Read the model definition and answer for the solid it produces. Units are mm, in the model's axes. A direction names the side the tool comes from. Round coordinates to 2 decimals unless told otherwise and drop trailing zeros. Order: outer loops, then holes, each group sorted by start corner. A loop starts at its lowest first (then second) coordinate and runs counter-clockwise, first axis right, second up.
from build123d import *
from build123d.topology import SkipClean

# Parameters (mm, degrees)
SKETCH1_R               = 1.8
MOUNTING_FACE_DEPTH     = 7.5
CELL_SUPPORT_FILLETS_R  = 7.5
MIDLINE_START           = 5
SKETCH3_W               = 20
SKETCH3_H               = 6
SKETCH3_R               = 1.8
SKETCH3_W_2             = 8
SKETCH3_H_2             = 9
MIDLINE_EXTENSION_DEPTH = 5


with BuildPart() as part:
    # Sketch1 → Mounting Face (new body)
    with BuildSketch(Plane.XY):
        Polygon((130, 0), (130, 9), (81.25, 9), (81.25, 44), (51.25, 44), (51.25, 9), (0, 9), (0, 0), align=None)
        with Locations((4, 3)):
            Circle(SKETCH1_R, mode=Mode.SUBTRACT)
        with Locations((61.25, 3)):
            Circle(SKETCH1_R, mode=Mode.SUBTRACT)
        with Locations((71.25, 3)):
            Circle(SKETCH1_R, mode=Mode.SUBTRACT)
        with Locations((125.75, 3)):
            Circle(SKETCH1_R, mode=Mode.SUBTRACT)
    extrude(amount=MOUNTING_FACE_DEPTH)

    # Cell Support Fillets
    cell_support_fillets_edges = [part.edges().sort_by_distance(p)[0] for p in [
        (51.25, 9, 3.75),
        (81.25, 9, 3.75),
    ]]
    fillet(cell_support_fillets_edges, radius=CELL_SUPPORT_FILLETS_R)

    # Sketch3 → Midline Extension (add)
    # profile 1 of 3: a face of its own
    with SkipClean():  # the faces are left unmerged after this step: merging them gives an invalid solid
        with BuildSketch(Plane(origin=(0, 0, 0), x_dir=(-1, 0, 0), z_dir=(0, 0, -1)).offset(MIDLINE_START)):
            with Locations((-66.25, 3)):
                Rectangle(SKETCH3_W, SKETCH3_H)
            with Locations((-71.25, 3)):
                Circle(SKETCH3_R, mode=Mode.SUBTRACT)
            with Locations((-61.25, 3)):
                Circle(SKETCH3_R, mode=Mode.SUBTRACT)
        # profile 2 of 3: a face of its own
        with BuildSketch(Plane(origin=(0, 0, 0), x_dir=(-1, 0, 0), z_dir=(0, 0, -1)).offset(MIDLINE_START)):
            with Locations((-4, 4.5)):
                Rectangle(SKETCH3_W_2, SKETCH3_H_2)
            with Locations((-4, 3)):
                Circle(SKETCH3_R, mode=Mode.SUBTRACT)
        # profile 3 of 3: a face of its own
        with BuildSketch(Plane(origin=(0, 0, 0), x_dir=(-1, 0, 0), z_dir=(0, 0, -1)).offset(MIDLINE_START)):
            with BuildLine():
                Line((-130, 0), (-124, 0))
                Line((-124, 0), (-124, 2.578692511))
                ThreePointArc((-124, 2.578692511), (-127.55, 3), (-124, 3.421307489))
                Line((-124, 3.421307489), (-124, 9))
                Line((-124, 9), (-130, 9))
                Line((-130, 9), (-130, 0))
            make_face()
        extrude(amount=-MIDLINE_EXTENSION_DEPTH)


solid = part.part
Q1. A cutting plane is placed at B-B, the plane x = 71.25. Give the vertices of the cut face in (y, z).
Outcome:
outline: (0, -5) - (1.2, -5) - (1.2, 7.5) - (0, 7.5) - close; (4.8, -5) - (6, -5) - (6, 0) - (44, 0) - (44, 7.5) - (4.8, 7.5) - close
Q2. A cutting plane is placed at D-D, the plane x = 58. Give the vertices of the cut face in (y, z), plus the area to 3 significant figures.
Outcome:
outline: (0, -5) - (6, -5) - (6, 0) - (44, 0) - (44, 7.5) - (0, 7.5) - close
area: 360 mm2
Q3. For faces 1 (the face through (81.25, 30, 4)), 2 (the face through (124, 6, -3)), 3 (the face through (51.25, 30, 4)), determine the directions among +Z, -Z, +X, -X, +Y, -Y from which every point of the face is accessible in a straight line to the end or side of a thin tool.
Outcome:
face 1: +Z, -Z, +X, +Y
face 2: -Z, +Y, -Y
face 3: +Z, -Z, -X, +Y
Q4. Straight lines are drawn through the part: probe 1 along Y at (x, z) = (4, -3.3); probe 2 along Y at (x, z) = (61.25, -2.1); probe 3 along Z at (x, y) = (29.5, 8.5). For each, find the intervals that lie inside material, in ascending order.
Outcome:
probe 1: y = 0 to 1.2, 4.8 to 9
probe 2: y = 0 to 1.2, 4.8 to 6
probe 3: z = 0 to 7.5
Q5. Flat-ended cylindrical pins translate along their axes: pin 1 (4 mm diameter, centred on x = 86, z = 6, fed in from +Y); pin 2 (2 mm diameter, centred on x = 91, y = 11.5, fed in from +Z); pin 3 (4 mm diameter, centred on x = 5, z = -2, fed in from +Y); pin 4 (6 mm diameter, centred on y = 24.5, z = 2.5, fed in from +X). Find the tip coordinate at first contact, or state that the pin passes through.
Outcome:
pin 1: stops at y = 10.7
pin 2: passes through
pin 3: stops at y = 9
pin 4: stops at x = 81.25
Q6. For a pull along X with two mould halves and no side action, classify faces 4 (the face through (66, 6, -3)), 5 (the face through (83.505, 11.139, 3.802)), 6 (the face through (66, 3, -5)) as released by +X, released by -X, zero draft, split by the parting line, or undercut.
Outcome:
face 4: undercut
face 5: released by +X
face 6: zero draft
Q7. A cutting plane is placed at C-C, the plane z = 3.5. Give the vertices of the cut face in (x, y), plus the area to 3 significant figures.
Outcome:
outline: (0, 0) - (130, 0) - (130, 9) - (88.75, 9) arc R7.5 cw to (81.25, 16.5) - (81.25, 44) - (51.25, 44) - (51.25, 16.5) arc R7.5 cw to (43.75, 9) - (0, 9) - close; hole circle Ø3.6 at (4, 3); hole circle Ø3.6 at (61.25, 3); hole circle Ø3.6 at (71.25, 3); hole circle Ø3.6 at (125.75, 3)
area: 2,200 mm2
